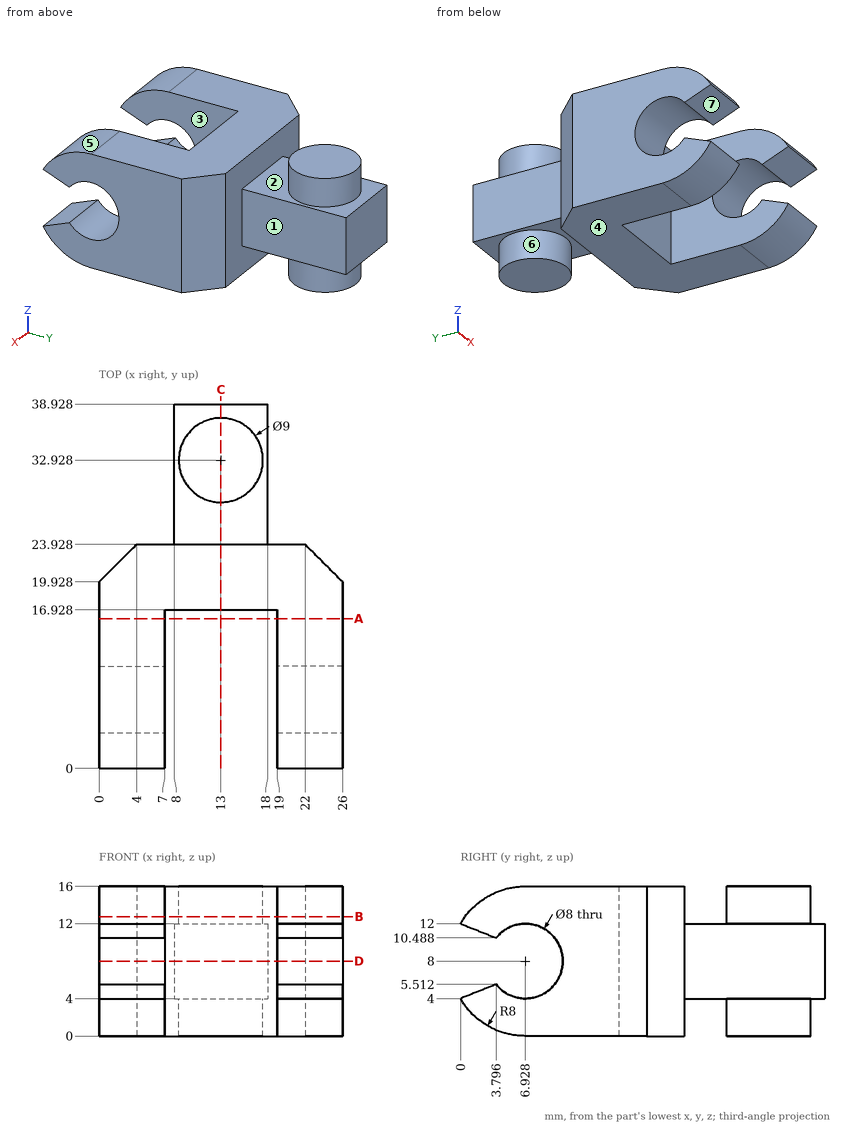
Could you check a few things on this drawing? It's one solid part, dimensions in mm from its lowest x, y, z. A direction names the side the tool comes from. Give positions to 0.01 mm unless a question says otherwise; leave off trailing zeros. Loops run counter-clockwise (first coordinate to the right, second up) from the corner with the lowest first, then second, coordinate; pieces in that order, holes last. Notation, with made-up numbers: (13, 18) -> (61, 18) arc R20 ccw to (61, 30) -> close; hole circle Ø1 at (76.5, -9). An arc over 180 degrees is marked (long way). Use one line per item in the form item = value. Start each with the question number.
1) Which directions (+Z, -Z, +X, -X, +Y, -Y) give clear straight access to the entire face, cutting with the end or side of a thin tool? Please do the marked faces 1, 2 and 3.
2) Thinking about a two-plate mould opening in Z: for the marked faces 4, 5, 6 and 7, which applies, +Z half, -Z half, draft (parallel to the pull), parting line (faces both ways), or undercut?
3) Imagine slicing it at B-B (z = 12.75). Please give me the cut outline in (x, y), then the cut area to 3 significant figures.
4) For P1, Ø5, axis at x = 15.5, z = 8, coming from the -Y side; P2, Ø2.5, axis at y = 28.5, z = 8, coming from the -X side; P3, Ø6, axis at x = 22.5, z = 4, coming from the +Y side, each with a flat end and sliding along its axis, tell me the tip position at first contact or that it passes through.
5) Imagine slicing it at C-C (x = 13). Please give me the cut outline in (y, z), then the cut area to 3 significant figures.
6) Please list where these lines run through material, in increasing order: line 1 along X through (y, z) = (14, 14); line 2 along Y through (x, z) = (16, 12.5) (1 decimal); line 3 along Z through (x, y) = (3.25, 8) (1 decimal).
7) Imagine slicing it at D-D (z = 8). Please give me the cut outline in (x, y).
8) Imagine slicing it at A-A (y = 16). Please give me the cut outline in (x, z), then the cut area to 3 significant figures.
Check values:
q1.face_1 = +Z, -Z, +X, +Y
q1.face_2 = +Z
q1.face_3 = +Z, -Z, -Y
q2.face_4 = -Z half
q2.face_5 = +Z half
q2.face_6 = draft
q2.face_7 = undercut
q3.outline = (0, 0.49) -> (7, 0.49) -> (7, 16.93) -> (19, 16.93) -> (19, 0.49) -> (26, 0.49) -> (26, 19.93) -> (22, 23.93) -> (4, 23.93) -> (0, 19.93) -> close; circle Ø9 at (13, 32.93)
q3.area = 460 mm^2
q4.P1 = 16.93
q4.P2 = 8
q4.P3 = 23.93
q5.outline = (16.93, 0) -> (23.93, 0) -> (23.93, 4) -> (28.43, 4) -> (28.43, 0) -> (37.43, 0) -> (37.43, 4) -> (38.93, 4) -> (38.93, 12) -> (37.43, 12) -> (37.43, 16) -> (28.43, 16) -> (28.43, 12) -> (23.93, 12) -> (23.93, 16) -> (16.93, 16) -> close
q5.area = 304 mm^2
q6.line_1 = 0 to 7, 19 to 26
q6.line_2 = 16.9 to 23.9, 29.6 to 36.3
q6.line_3 = 0 to 4.1, 11.9 to 16
q7.outline = (0, 10.93) -> (7, 10.93) -> (7, 16.93) -> (19, 16.93) -> (19, 10.93) -> (26, 10.93) -> (26, 19.93) -> (22, 23.93) -> (18, 23.93) -> (18, 38.93) -> (8, 38.93) -> (8, 23.93) -> (4, 23.93) -> (0, 19.93) -> close
q8.outline = (0, 0) -> (7, 0) -> (7, 16) -> (0, 16) -> close; (19, 0) -> (26, 0) -> (26, 16) -> (19, 16) -> close
q8.area = 224 mm^2
